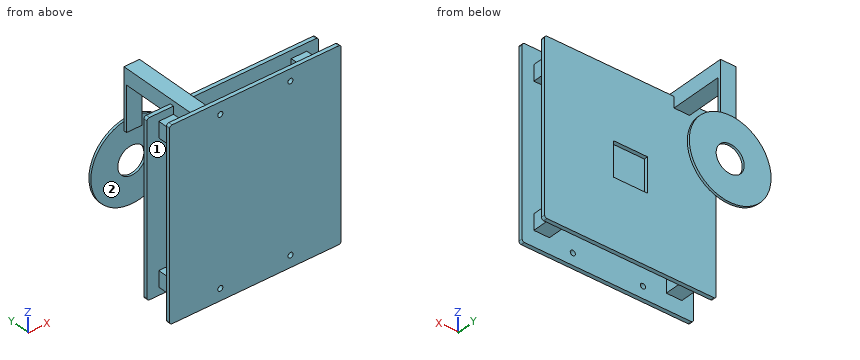
```python
from build123d import *

# Parameters (mm, degrees)
BASE_PLATE_PROFILE_W       = 220
BASE_PLATE_PROFILE_H       = 240
BASE_PLATE_DEPTH           = 5
STANDOFFS_START            = 5
STANDOFFS_PROFILE_W        = 20
STANDOFFS_PROFILE_H        = 20
STANDOFFS_DEPTH            = 30
HOLDER_START               = 35
HOLDER_SEAT_PROFILE_W      = 220
HOLDER_SEAT_PROFILE_H      = 220
HOLDER_SEAT_PROFILE_W_2    = 44
HOLDER_SEAT_PROFILE_H_2    = 44
HOLDER_SEAT_DEPTH          = 5
GUIDE_START                = 5
GUIDE_COLUMN_PROFILE_W     = 20
GUIDE_COLUMN_PROFILE_H     = 20
GUIDE_COLUMN_DEPTH         = 107
GUIDE_START_2              = 108
GUIDE_ARM_PROFILE_W        = 20
GUIDE_ARM_PROFILE_H        = 77.313861244
GUIDE_ARM_DEPTH            = 4
GUIDE_START_3              = 112
GUIDE_SEAT_PROFILE_R       = 52.5
GUIDE_SEAT_PROFILE_R_2     = 18
GUIDE_SEAT_DEPTH           = 3
BASE_START                 = 2.5
BASE_FIXING_HOLES_LAYOUT_R = 3.3
BASE_FIXING_HOLES_DEPTH    = 2.5
PLATE_CORNER_RADII_R       = 3


with BuildPart() as part:
    # Base Plate Profile → Base Plate (new body)
    with BuildSketch(Plane(origin=(0, 0, 0), x_dir=(1, 0, 0), z_dir=(0, 1, 0))):
        Rectangle(BASE_PLATE_PROFILE_W, BASE_PLATE_PROFILE_H)
    extrude(amount=BASE_PLATE_DEPTH)

    # Standoffs Profile → Standoffs (add)
    with BuildSketch(Plane(origin=(0, 0, 0), x_dir=(1, 0, 0), z_dir=(0, 1, 0)).offset(STANDOFFS_START)):
        with Locations((-85, 90)):
            Rectangle(STANDOFFS_PROFILE_W, STANDOFFS_PROFILE_H)
        with Locations((-85, -90)):
            Rectangle(STANDOFFS_PROFILE_W, STANDOFFS_PROFILE_H)
        with Locations((85, 90)):
            Rectangle(STANDOFFS_PROFILE_W, STANDOFFS_PROFILE_H)
        with Locations((85, -90)):
            Rectangle(STANDOFFS_PROFILE_W, STANDOFFS_PROFILE_H)
    extrude(amount=STANDOFFS_DEPTH)

    # Holder Seat Profile → Holder Seat (add)
    with BuildSketch(Plane(origin=(0, 0, 0), x_dir=(1, 0, 0), z_dir=(0, 1, 0)).offset(HOLDER_START)):
        Rectangle(HOLDER_SEAT_PROFILE_W, HOLDER_SEAT_PROFILE_H)
        Rectangle(HOLDER_SEAT_PROFILE_W_2, HOLDER_SEAT_PROFILE_H_2, mode=Mode.SUBTRACT)
    extrude(amount=HOLDER_SEAT_DEPTH)

    # Guide Column Profile → Guide Column (add)
    with BuildSketch(Plane(origin=(0, 0, 0), x_dir=(1, 0, 0), z_dir=(0, 1, 0)).offset(GUIDE_START)):
        with Locations((-65.986921194, -106)):
            Rectangle(GUIDE_COLUMN_PROFILE_W, GUIDE_COLUMN_PROFILE_H)
    extrude(amount=GUIDE_COLUMN_DEPTH)

    # Guide Arm Profile → Guide Arm (add)
    with BuildSketch(Plane(origin=(0, 0, 0), x_dir=(1, 0, 0), z_dir=(0, 1, 0)).offset(GUIDE_START_2)):
        with Locations((-65.986921194, -77.343069378)):
            Rectangle(GUIDE_ARM_PROFILE_W, GUIDE_ARM_PROFILE_H)
    extrude(amount=GUIDE_ARM_DEPTH)

    # Guide Seat Profile → Guide Seat (add)
    with BuildSketch(Plane(origin=(0, 0, 0), x_dir=(1, 0, 0), z_dir=(0, 1, 0)).offset(GUIDE_START_3)):
        with Locations(Location((-65.986921194, 1.313861244, 0), (0, 0, 259.019424572))):
            Circle(GUIDE_SEAT_PROFILE_R)
        with Locations(Location((-65.986921194, 1.313861244, 0), (0, 0, 270))):
            Circle(GUIDE_SEAT_PROFILE_R_2, mode=Mode.SUBTRACT)
    extrude(amount=GUIDE_SEAT_DEPTH)

    # Base Fixing Holes Layout → Base Fixing Holes (cut, symmetric)
    with BuildSketch(Plane(origin=(0, 0, 0), x_dir=(1, 0, 0), z_dir=(0, 1, 0)).offset(BASE_START)):
        with Locations(Location((-45, 105, 0), (0, 0, 270))):
            Circle(BASE_FIXING_HOLES_LAYOUT_R)
        with Locations(Location((-45, -105, 0), (0, 0, 270))):
            Circle(BASE_FIXING_HOLES_LAYOUT_R)
        with Locations(Location((45, 105, 0), (0, 0, 270))):
            Circle(BASE_FIXING_HOLES_LAYOUT_R)
        with Locations(Location((45, -105, 0), (0, 0, 270))):
            Circle(BASE_FIXING_HOLES_LAYOUT_R)
    extrude(amount=BASE_FIXING_HOLES_DEPTH, both=True, mode=Mode.SUBTRACT)

    # Plate Corner Radii
    plate_corner_radii_edges = [part.edges().sort_by_distance(p)[0] for p in [
        (-110, 37.5, -110),
        (-110, 37.5, 110),
        (110, 37.5, 110),
        (110, 37.5, -110),
        (-110, 2.5, -120),
        (110, 2.5, -120),
        (110, 2.5, 120),
        (-110, 2.5, 120),
    ]]
    fillet(plate_corner_radii_edges, radius=PLATE_CORNER_RADII_R)


solid = part.part
```
The model under review builds one solid part; all positions refer to its coordinate system, in mm. Face numbers are marked on the shaded views. Give positions to 0.01 mm unless a question says otherwise; leave off trailing zeros. Write each loop counter-clockwise with the first axis right and the second up, starting at its lowest first coordinate (ties: lowest second). Pieces come first, ordered by that corner, then holes. Notation, with made-up numbers: (34, 25.25) -> (42, 25.25) arc R23 ccw to (42, 46.25) -> close; hole circle Ø7 at (25.5, 5.5). An arc over 180 degrees is marked (long way). Answer in a Markdown table with one row per item.
1) Mouldability with a two-part tool opening along X and no side actions: class the marked faces 1 and 2 as +X half, -X half, draft (parallel to the pull), parting line (faces both ways), or undercut.
Worked answers:
| item | result |
|---|---|
| face 1 | undercut |
| face 2 | draft |
2) For L1, parallel to X at y = 1.7, z = 105; L2, parallel to Y at x = -62, z = 76.5; L3, parallel to Y at x = -20.5, z = 66, list the stretches that pass through material, from the lowest coordinate up. Write a range as [from, to].
Worked answers:
| item | result |
|---|---|
| L1 | [-110, -48.3], [-41.7, 41.7], [48.3, 110] |
| L2 | [0, 5], [35, 40], [108, 112] |
| L3 | [0, 5], [35, 40] |
3) Add section B-B on z = 59.5. State the section outline as (x, y) points, plus the area to 3 significant figures.
Worked answers:
| item | result |
|---|---|
| outline | (-110, 0) -> (110, 0) -> (110, 5) -> (-110, 5) -> close; (-110, 35) -> (110, 35) -> (110, 40) -> (-110, 40) -> close; (-75.99, 108) -> (-55.99, 108) -> (-55.99, 112) -> (-75.99, 112) -> close |
| area | 2,280 mm² |
4) Add section C-C on x = 4. State the section outline as (y, z) points.
Worked answers:
| item | result |
|---|---|
| outline | (0, -120) -> (5, -120) -> (5, 120) -> (0, 120) -> close; (35, -110) -> (40, -110) -> (40, -22) -> (35, -22) -> close; (35, 22) -> (40, 22) -> (40, 110) -> (35, 110) -> close |
5) Add section D-D on y = 9.5. State the section outline as (x, z) points.
Worked answers:
| item | result |
|---|---|
| outline | (-95, -100) -> (-75, -100) -> (-75, -80) -> (-95, -80) -> close; (-95, 80) -> (-75, 80) -> (-75, 96) -> (-55.99, 96) -> (-55.99, 116) -> (-75.99, 116) -> (-75.99, 100) -> (-95, 100) -> close; (75, -100) -> (95, -100) -> (95, -80) -> (75, -80) -> close; (75, 80) -> (95, 80) -> (95, 100) -> (75, 100) -> close |
6) Add section A-A on x = 45. State the section outline as (y, z) points, plus the area to 3 significant figures.
Worked answers:
| item | result |
|---|---|
| outline | (0, -120) -> (5, -120) -> (5, -108.3) -> (0, -108.3) -> close; (0, -101.7) -> (5, -101.7) -> (5, 101.7) -> (0, 101.7) -> close; (0, 108.3) -> (5, 108.3) -> (5, 120) -> (0, 120) -> close; (35, -110) -> (40, -110) -> (40, 110) -> (35, 110) -> close |
| area | 2,230 mm² |
7) Clearance check with flat-ended pins moving along their axes: P1, Ø2.5, axis at x = -4.5, y = 36.5, coming from the -Z side; P2, Ø6, axis at y = 20, z = 89.5, coming from the -X side; P3, Ø12, axis at y = 32, z = 2, coming from the -X side. State where each tip first meets the part, or that it passes through.
Worked answers:
| item | result |
|---|---|
| P1 | z = -110 |
| P2 | x = -95 |
| P3 | x = -110 |
